Can you work these out from the model? Positions are in its coordinate system, mm. Round coordinates to 2 decimals unless told otherwise and drop trailing zeros. Loops run counter-clockwise (first coordinate to the right, second up) from the corner with the lowest first, then second, coordinate; pieces in that order, holes last. Notation, with made-up numbers: (18.25, 12.25) - (23.25, 12.25) arc R22 cw to (23.25, 46.25) - close; hole circle Ø6 at (9, 76.5). An arc over 180 degrees is marked (long way). Answer as CSV lines item,"result".
Autodesk Inventor part; units mm, degrees
sketch "Boceto1" plane through (0, 0, 0) normal (0, 0, 1) x (1, 0, 0)
  line L0 (-75, 75) -> (75, 75)
  line L1 (75, 75) -> (75, -75)
  line L2 (75, -75) -> (-75, -75)
  line L3 (-75, -75) -> (-75, 75)
  line L4 (-75, 75) -> (75, -75) construction
  line L5 (75, 75) -> (-75, -75) construction
  point P0 (0, 0)
  dimension "d0" = 150
  dimension "d1" = 150
extrude "Extrusión1" add sketch "Boceto1" along normal blind 25.4
sketch "Boceto3" plane through (0, 0, 0) normal (0, 1, 0) x (-1, 0, 0)
  line L0 (-75, 25.4) -> (75, 25.4)
  arc A0 (-15, 25.4) -> (15, 25.4) centre (0, 25.4) ccw
  line L1 (15, 25.4) -> (-15, 25.4)
  point P0 (0, 0)
  dimension "d7" = 15
revolve "Revolución2" cut sketch "Boceto3" angle 360 about axis through (75, 0, 25.4) along (-1, 0, 0)
ref_plane "Plano de trabajo1" through (-75, -75, 0) normal (-0.7071068, 0.7071068, 0) x (0, 0, 1)
ref_plane "Plano de trabajo2" through (75, -75, 0) normal (-0.7071068, -0.7071068, 0) x (0, 0, 1)
sketch "Boceto4" plane through (-75, -75, 0) normal (-0.7071068, 0.7071068, 0) x (0, 0, 1)
  line L0 (25.4, 106.066) -> (25.4, 0)
  arc A0 (25.4, 68.9087) -> (25.4, 48.9087) centre (25.4, 58.9087) ccw
  line L1 (25.4, 48.9087) -> (25.4, 68.9087)
  point P0 (0, 106.066)
  dimension "d11" = 10
sketch "Boceto5" plane through (75, -75, 0) normal (-0.7071068, -0.7071068, 0) x (0, 0, 1)
  line L0 (25.4, 106.066) -> (25.4, 212.132)
  arc A0 (25.4, 171.8235) -> (25.4, 147.8235) centre (25.4, 159.8235) ccw
  line L1 (25.4, 171.8235) -> (25.4, 147.8235)
  point P0 (0, 106.066)
  dimension "d12" = 12
sketch "Boceto6" plane through (0, 0, 0) normal (0, 1, 0) x (-1, 0, 0)
  arc A0 (-55.646, 25.4) -> (-19.646, 25.4) centre (-37.646, 25.4) ccw
  line L0 (-19.646, 25.4) -> (-55.646, 25.4)
  line L1 (-75, 25.4) -> (75, 25.4)
  point P0 (0, 0)
  dimension "d13" = 18
revolve "Revolución3" cut sketch "Boceto5" angle 360 about axis through (0, 0, 25.4) along (-0.7071068, 0.7071068, 0)
revolve "Revolución4" cut sketch "Boceto4" angle 360 about axis through (0, 0, 25.4) along (-0.7071068, -0.7071068, 0)
revolve "Revolución5" cut sketch "Boceto6" angle 360 about axis through (19.646, 0, 25.4) along (1, 0, 0)
properties part number "Placa - Pitting Esfera"
Q1. If I drill on line 1 along X through (y, z) = (-9, 19.75); line 2 along Y through (x, z) = (-40.5, 14.75); line 3 along X through (y, z) = (-6, 10), over which ranges is the centre line in solid material (lowest first)? Write a range as [from, to].
Checks:
line 1,"[-75, -10.59], [10.59, 23.12], [52.17, 75]"
line 2,"[-75, 33.07], [42.95, 75]"
line 3,"[-75, 30.52], [44.78, 75]"
Q2. Imagine slicing it at A-A (z = 22.75). Write out the boundary of the cut face in (x, y).
Checks:
outline,"(-75, -75) - (75, -75) - (75, 75) - (-75, 75) - close; hole circle Ø23.41 at (-38.01, 38.01); hole circle Ø19.28 at (-33.35, -33.35); hole circle Ø29.53 at (0, 0); hole circle Ø35.61 at (37.65, 0)"
Q3. Imagine slicing it at B-B (x = 51.5). Write out the boundary of the cut face in (y, z).
Checks:
outline,"(-75, 0) - (75, 0) - (75, 25.4) - (11.49, 25.4) arc R11.49 cw to (-11.49, 25.4) - (-75, 25.4) - close"
Q4. Imagine slicing it at C-C (y = -8). Write out the boundary of the cut face in (x, z).
Checks:
outline,"(-75, 0) - (75, 0) - (75, 25.4) - (53.77, 25.4) arc R16.12 cw to (21.52, 25.4) - (12.69, 25.4) arc R12.69 cw to (-12.69, 25.4) - (-75, 25.4) - close"
Q5. I'm going to push a flat-ended pin straight in: pin 1 Ø2 at (x, y) = (29.5, -7.5) entering from +Z. Where does the tip first touch, or does it pass through?
Checks:
pin 1,"z = 12.05"
Q6. Imagine slicing it at D-D (x = -1). Write out the boundary of the cut face in (y, z).
Checks:
outline,"(-75, 0) - (75, 0) - (75, 25.4) - (14.97, 25.4) arc R14.97 cw to (-14.97, 25.4) - (-75, 25.4) - close"
